from build123d import *

# Parameters (mm, degrees)
F1_DEPTH = 9.525
F2_R     = 1.98374
F3_R     = 3.69316
F4_R     = 1.35255
F5_DEPTH = 108.98632
F6_R     = 1.35255
F6_R_2   = 3.175
F7_DEPTH = 1.70942
F8_R     = 0.762


with BuildPart() as f1:
    # F0 (on Top) → F1 (new body)
    with BuildSketch(Plane.XY):
        Polygon((0, 25.4), (0, 0), (-105.56748, 0), (-105.56748, 25.4), (-107.2769, 25.4), (-107.2769, -1.70942), (1.70942, -1.70942), (1.70942, 25.4), align=None)
    extrude(amount=F1_DEPTH)

    # F2
    f2_edges = [f1.edges().sort_by_distance(p)[0] for p in [
        (0, 0, 4.7625),
        (-105.56748, 0, 4.7625),
    ]]
    fillet(f2_edges, radius=F2_R)

    # F3
    f3_edges = [f1.edges().sort_by_distance(p)[0] for p in [
        (1.70942, -1.70942, 4.7625),
        (-107.2769, -1.70942, 4.7625),
    ]]
    fillet(f3_edges, radius=F3_R)

    # F4 (on face) → F5 (cut, through all)
    with BuildSketch(Plane(origin=(-107.2769, 0, 0), x_dir=(0, -1, 0), z_dir=(-1, 0, 0))):
        with Locations((-20.6375, 4.7625)):
            Circle(F4_R)
        with Locations((-6.74624, 4.7625)):
            Circle(F4_R)
    extrude(amount=-F5_DEPTH, mode=Mode.SUBTRACT)

    # F6 (on face) → F7 (cut, through all)
    with BuildSketch(Plane.XZ.offset(1.70942)):
        with Locations((-98.82124, 4.7625)):
            Circle(F6_R)
        with Locations((-6.74624, 4.7625)):
            Circle(F6_R)
        with Locations((-67.8351831, 4.7625)):
            Circle(F6_R)
        with Locations((-37.7322969, 4.7625)):
            Circle(F6_R)
        with Locations((-52.78374, 4.7625)):
            Circle(F6_R_2)
    extrude(amount=-F7_DEPTH, mode=Mode.SUBTRACT)

    # F8
    f8_edges = [f1.edges().sort_by_distance(p)[0] for p in [
        (-106.42219, 25.4, 9.525),
        (-106.42219, 25.4, 0),
        (0.85471, 25.4, 9.525),
        (0.85471, 25.4, 0),
    ]]
    fillet(f8_edges, radius=F8_R)


solid = f1.part
For this review, take the finished solid that the model builds, in its own axes (mm). A direction names the side the tool comes from. Round coordinates to 2 decimals unless told otherwise and drop trailing zeros. Loops run counter-clockwise (first coordinate to the right, second up) from the corner with the lowest first, then second, coordinate; pieces in that order, holes last. Notation, with made-up numbers: (26.5, -1) - (54.5, -1) arc R15 ccw to (54.5, 11) - close; hole circle Ø5 at (85.25, 52). An arc over 180 degrees is marked (long way). Put each result on its own line as item: value. Start each with the question number.
1. Insertion check: P1, Ø1, axis at x = -47, z = 2.5, coming from the +Y side. The pin has a flat end and moves straight along its axis. Give the tip position at first contact, or say it passes through.
2. Mouldability with a two-part tool opening along X and no side actions: class faces 1 (the cylindrical face through (-106.434, 19.347, 5.169)), 2 (the cylindrical face through (0.656, -0.599, 4.829)), 3 (the flat face through (-52, 0, 8)) as +X half, -X half, draft (parallel to the pull), parting line (faces both ways), or undercut.
3. Consider section C-C on z = 2.5. State the section outline as (x, y) points, plus the area to 3 significant figures.
4. Consider section B-B on x = -52. State the section outline as (y, z) points (3 decimals).
5. Consider section A-A on y = 16.5. State the section outline as (x, z) points (3 decimals), plus the area to 3 significant figures.
6. Consider section D-D on x = -12. State the section outline as (y, z) points (3 decimals).
7. For faces 4 (the flat face through (-105.567, 14, 5)), 5 (the cylindrical face through (-106.43, 7.74, 5.68)), list the 3-axis set-ups (+Z, -Z, +X, -X, +Y, -Y) from which the entire face can be reached by the end or side of a thin tool; tool diameter is ignored.
8. For probe 1 along X at (y, z) = (6, 3); probe 2 along Y at (x, z) = (-15.5, 5.25), list the stretches that pass through material, from the lowest coordinate up. Write a range as [from, to].
Result sheet:
1. P1: y = 0
2. face 1: draft
2. face 2: +X half
2. face 3: undercut
3. outline: (-107.28, 1.98) arc R3.69 ccw to (-103.58, -1.71) - (-55.01, -1.71) - (-55.01, 0) - (-103.58, 0) arc R1.98 cw to (-105.57, 1.98) - (-105.57, 25.4) - (-107.28, 25.4) - close; (-50.56, -1.71) - (-1.98, -1.71) arc R3.69 ccw to (1.71, 1.98) - (1.71, 25.4) - (0, 25.4) - (0, 1.98) arc R1.98 cw to (-1.98, 0) - (-50.56, 0) - close
3. area: 261 mm^2
4. outline: (-1.709, 0) - (0, 0) - (0, 1.686) - (-1.709, 1.686) - close; (-1.709, 7.839) - (0, 7.839) - (0, 9.525) - (-1.709, 9.525) - close
5. outline: (-107.277, 0) - (-105.567, 0) - (-105.567, 9.525) - (-107.277, 9.525) - close; (0, 0) - (1.709, 0) - (1.709, 9.525) - (0, 9.525) - close
5. area: 32.6 mm^2
6. outline: (-1.709, 0) - (0, 0) - (0, 9.525) - (-1.709, 9.525) - close
7. face 4: +Z, -Z, +Y
7. face 5: +X, -X
8. probe 1: [-107.28, -105.57], [0, 1.71]
8. probe 2: [-1.71, 0]
